from build123d import *

# Parameters (mm, degrees)
BOSS_EXTRUDE1_DEPTH = 4.7625


with BuildPart() as part:
    # Sketch2 → Boss-Extrude1 (new body)
    with BuildSketch(Plane.XY):
        with BuildLine():
            Line((64.13459107, 7.698729744), (38.73459107, 51.692820256))
            ThreePointArc((38.73459107, 51.692820256), (33.098729744, 57.328681582), (25.4, 59.39155))
            Line((25.4, 59.39155), (-25.4, 59.39155))
            ThreePointArc((-25.4, 59.39155), (-33.098729744, 57.328681582), (-38.73459107, 51.692820256))
            Line((-38.73459107, 51.692820256), (-64.13459107, 7.698729744))
            ThreePointArc((-64.13459107, 7.698729744), (-66.197459488, 0), (-64.13459107, -7.698729744))
            Line((-64.13459107, -7.698729744), (-38.73459107, -51.692820256))
            ThreePointArc((-38.73459107, -51.692820256), (-33.098729744, -57.328681582), (-25.4, -59.39155))
            Line((-25.4, -59.39155), (25.4, -59.39155))
            ThreePointArc((25.4, -59.39155), (33.098729744, -57.328681582), (38.73459107, -51.692820256))
            Line((38.73459107, -51.692820256), (64.13459107, -7.698729744))
            ThreePointArc((64.13459107, -7.698729744), (66.197459488, 0), (64.13459107, 7.698729744))
        make_face()
    extrude(amount=BOSS_EXTRUDE1_DEPTH)


solid = part.part
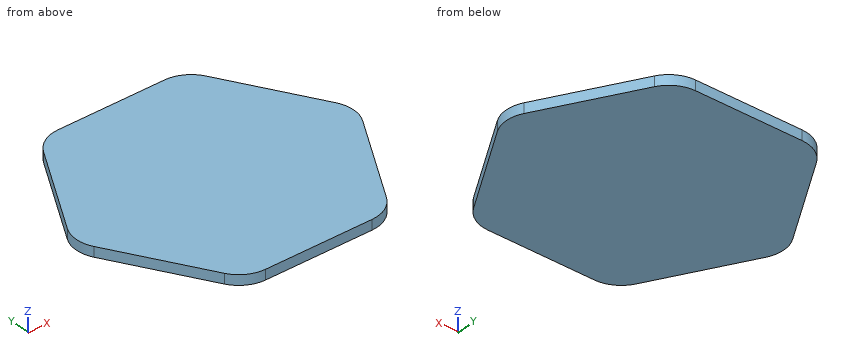
Work out the finished part from the listing and answer in its coordinate system (mm). Round coordinates to 2 decimals unless told otherwise and drop trailing zeros. Write each loop counter-clockwise with the first axis right and the second up, starting at its lowest first coordinate (ties: lowest second). Pieces come first, ordered by that corner, then holes. Notation, with made-up numbers: M 43,-30.75 L 66,-30.75 A4 ccw 66,-26.75 Z; hole C -3,36 d3. An arc over 180 degrees is marked long. Use a Markdown table: item, result.
1) Flat-ended cylindrical pins translate along their axes: pin 1 (1 mm diameter, centred on y = 8.5, z = 1, fed in from +X); pin 2 (1.5 mm diameter, centred on x = 30.5, y = -22.5, fed in from -Z). Find the tip coordinate at first contact, or state that the pin passes through.
Taken from the geometry:
| item | result |
|---|---|
| pin 1 | stops at x = 63.96 |
| pin 2 | stops at z = 0 |
2) The part is cut by section B-B on x = -49.5. Give the vertices of the cut face in (y, z).
Taken from the geometry:
| item | result |
|---|---|
| outline | M -33.05,0 L 33.05,0 L 33.05,4.76 L -33.05,4.76 Z |
3) Consider line 1 (X direction, y = -41.5, z = 0.85); line 2 (Y direction, x = 29, z = 2.3); line 3 (X direction, y = 47, z = 0.8). Determine where each line is inside the solid, lowest interval first. Write a range as [from, to].
Taken from the geometry:
| item | result |
|---|---|
| line 1 | x = [-44.62, 44.62] |
| line 2 | y = [-58.96, 58.96] |
| line 3 | x = [-41.44, 41.44] |
4) The part is cut by section A-A on z = 1.45. Give the vertices of the cut face in (x, y).
Taken from the geometry:
| item | result |
|---|---|
| outline | M -64.13,-7.7 L -38.73,-51.69 A15.4 ccw -25.4,-59.39 L 25.4,-59.39 A15.4 ccw 38.73,-51.69 L 64.13,-7.7 A15.4 ccw 64.13,7.7 L 38.73,51.69 A15.4 ccw 25.4,59.39 L -25.4,59.39 A15.4 ccw -38.73,51.69 L -64.13,7.7 A15.4 ccw Z |
5) The part is cut by section C-C on y = -15. Give the vertices of the cut face in (x, z), plus the area to 3 significant figures.
Taken from the geometry:
| item | result |
|---|---|
| outline | M -59.92,0 L 59.92,0 L 59.92,4.76 L -59.92,4.76 Z |
| area | 571 mm2 |
